The listing builds one solid part. Answer for the finished solid, in the listing's coordinates (mm). Coordinates: 2 decimals unless noted, no trailing zeros. Order: outer loops, then holes, each group sorted by start corner. A loop starts at its lowest first (then second) coordinate and runs counter-clockwise, first axis right, second up.
Autodesk Inventor part; units mm, degrees
ref_plane "YZ Plane" through (0, 0, 0) normal (1, 0, 0) x (0, 1, 0)
ref_plane "XZ Plane" through (0, 0, 0) normal (0, 1, 0) x (-1, 0, 0)
ref_plane "XY Plane" through (0, 0, 0) normal (0, 0, 1) x (1, 0, 0)
sketch "Sketch1" plane through (0, 0, 0) normal (1, 0, 0) x (0, 1, 0)
  line L0 (0, 0) -> (3, 0)
  line L1 (3, 0) -> (3, -87.28)
  line L2 (3, -87.28) -> (0, -87.28)
  line L3 (0, -87.28) -> (0, 0)
  line L4 (3.125, -87.405) -> (3.125, 0.125)
  line L5 (3.125, 0.125) -> (-0.125, 0.125)
  line L6 (-0.125, 0.125) -> (-0.125, -87.405)
  line L7 (-0.125, -87.405) -> (3.125, -87.405)
  line L8 (5.125, 2.125) -> (5.125, -89.405)
  line L9 (5.125, -89.405) -> (-2.125, -89.405)
  line L10 (-2.125, -89.405) -> (-2.125, 2.125)
  line L11 (-2.125, 2.125) -> (5.125, 2.125)
  line L12 (3, -87.28) -> (15, -87.28)
  line L13 (15, -87.28) -> (15, -84.28)
  line L14 (15, -84.28) -> (3, -84.28)
  line L15 (3, -84.28) -> (3, -87.28)
  line L16 (3, 0) -> (15, 0)
  line L17 (15, 0) -> (15, -3)
  line L18 (15, -3) -> (3, -3)
  line L19 (3, -3) -> (3, 0)
  line L20 (15.1, 0.1) -> (2.9, 0.1)
  line L21 (2.9, 0.1) -> (2.9, -3.1)
  line L22 (2.9, -3.1) -> (15.1, -3.1)
  line L23 (15.1, -3.1) -> (15.1, 0.1)
  line L24 (15.1, -87.38) -> (2.9, -87.38)
  line L25 (2.9, -87.38) -> (2.9, -84.18)
  line L26 (2.9, -84.18) -> (15.1, -84.18)
  line L27 (15.1, -84.18) -> (15.1, -87.38)
  line L28 (0.875, -89.405) -> (17.125, -89.405)
  line L29 (17.125, -89.405) -> (17.125, -82.155)
  line L30 (17.125, -82.155) -> (0.875, -82.155)
  line L31 (0.875, -82.155) -> (0.875, -89.405)
  line L32 (17.125, 2.125) -> (0.875, 2.125)
  line L33 (0.875, 2.125) -> (0.875, -5.125)
  line L34 (0.875, -5.125) -> (17.125, -5.125)
  line L35 (17.125, -5.125) -> (17.125, 2.125)
  line L36 (15.1, 0.1) -> (17.125, 0.1)
  line L37 (15.1, -3.1) -> (17.125, -3.1)
  line L38 (15.1, -87.38) -> (17.125, -87.38)
  line L39 (15.1, -84.18) -> (17.125, -84.18)
  point P0 (5.125, -82.155)
  point P1 (5.125, -5.125)
  point P2 (3.125, -84.18)
  point P3 (3.125, -87.38)
  point P4 (3.125, 0.1)
  point P5 (3.125, -3.1)
  dimension "d0" = 87.28
  dimension "d1" = 3
  dimension "d2" = 0.125
  dimension "d3" = 2
  dimension "d4" = 12
  dimension "d5" = 3
  dimension "d6" = 12
  dimension "d7" = 3
  dimension "d8" = 0.1
  dimension "d9" = 0.1
  dimension "d10" = 0
  dimension "d11" = 0
extrude "Extrusion1" add sketch "Sketch1" along normal blind 6.5 contours L33 L11 L8 L20 L4 L5 | L5 L6 L7 L31 L9 L10 L11 L33 | L7 L4 L24 L8 L9 L31 | L32 L35 L36 L20 L8 | L34 L8 L30 L4 | L4 L22 L8 L34 | L30 L8 L26 L4 | L8 L22 L37 L35 L34 | L8 L24 L38 L29 L28 | L30 L29 L39 L26 L8
sketch "Sketch2" plane through (6.5, 0, 0) normal (1, 0, 0) x (0, 0, -1)
  line L0 (3.1, 16.125) -> (-0.1, 16.125)
  line L1 (-0.1, 16.125) -> (-0.1, 3.325)
  line L2 (-0.1, 3.325) -> (3.1, 3.325)
  line L3 (3.1, 3.325) -> (3.1, 16.125)
  line L4 (3.1, 3.125) -> (84.18, 3.125)
  line L5 (5.125, 17.125) -> (3.1, 17.125)
  line L6 (-0.1, 3.125) -> (-0.1, 17.125)
  line L7 (3.1, 17.125) -> (3.1, 3.125)
  line L8 (84.18, 3.325) -> (87.38, 3.325)
  line L9 (87.38, 3.325) -> (87.38, 16.125)
  line L10 (87.38, 16.125) -> (84.18, 16.125)
  line L11 (84.18, 16.125) -> (84.18, 3.325)
  line L12 (89.405, 17.125) -> (87.38, 17.125)
  line L13 (87.38, 17.125) -> (87.38, 3.125)
  line L14 (84.18, 3.125) -> (84.18, 17.125)
  line L15 (28.765, -0.125) -> (58.515, -0.125)
  line L16 (58.515, -0.125) -> (58.515, 3.125)
  line L17 (58.515, 3.125) -> (28.765, 3.125)
  line L18 (28.765, 3.125) -> (28.765, -0.125)
  line L19 (87.405, -0.125) -> (-0.125, -0.125)
  line L20 (-0.125, -0.125) -> (-0.125, 3.125)
  point P0 (0, 0)
  dimension "d14" = 0.2
  dimension "d15" = 1
  dimension "d16" = 0
  dimension "d17" = 0
  dimension "d18" = 0.2
  dimension "d19" = 1
  dimension "d20" = 0
  dimension "d21" = 0
  dimension "d22" = 29.75
  dimension "d23" = 0
  dimension "d24" = 0
  dimension "d25" = 28.89
extrude "Extrusion2" add sketch "Sketch2" against normal blind 2.85
sketch "Sketch3" plane through (6.5, 0, 0) normal (1, 0, 0) x (0, 0, -1)
  line L0 (84.18, 16.125) -> (84.18, 17.125)
  line L1 (84.18, 17.125) -> (82.155, 17.125)
  line L2 (82.155, 17.125) -> (82.155, 5.125)
  line L3 (82.155, 5.125) -> (5.125, 5.125)
  line L4 (5.125, 5.125) -> (5.125, 17.125)
  line L5 (5.125, 17.125) -> (3.1, 17.125)
  line L6 (3.1, 17.125) -> (3.1, 16.125)
  line L7 (3.1, 16.125) -> (-0.1, 16.125)
  line L8 (-0.1, 16.125) -> (-0.1, 17.125)
  line L9 (-0.1, 17.125) -> (-2.125, 17.125)
  line L10 (-2.125, 17.125) -> (-2.125, -2.125)
  line L11 (-2.125, -2.125) -> (89.405, -2.125)
  line L12 (89.405, -2.125) -> (89.405, 17.125)
  line L13 (89.405, 17.125) -> (87.38, 17.125)
  line L14 (87.38, 17.125) -> (87.38, 16.125)
  line L15 (87.38, 16.125) -> (84.18, 16.125)
  line L16 (84.18, 3.325) -> (87.38, 3.325)
  line L17 (87.38, 3.325) -> (87.38, 3.125)
  line L18 (87.38, 3.125) -> (87.405, 3.125)
  line L19 (87.405, 3.125) -> (87.405, -0.125)
  line L20 (87.405, -0.125) -> (58.515, -0.125)
  line L21 (58.515, -0.125) -> (58.515, 3.125)
  line L22 (58.515, 3.125) -> (84.18, 3.125)
  line L23 (84.18, 3.125) -> (84.18, 3.325)
  line L24 (28.765, 3.125) -> (28.765, -0.125)
  line L25 (28.765, -0.125) -> (-0.125, -0.125)
  line L26 (-0.125, -0.125) -> (-0.125, 3.125)
  line L27 (-0.125, 3.125) -> (-0.1, 3.125)
  line L28 (-0.1, 3.125) -> (-0.1, 3.325)
  line L29 (-0.1, 3.325) -> (3.1, 3.325)
  line L30 (3.1, 3.325) -> (3.1, 3.125)
  line L31 (3.1, 3.125) -> (28.765, 3.125)
  point P0 (0, 0)
extrude "Extrusion4" add sketch "Sketch3" along normal blind 2.5 contours L15 L14 L13 L12 L11 L10 L9 L8 L7 L6 L5 L4 L3 L2 L1 L0 | L16 L17 L18 L19 L20 L21 L22 L23 | L24 L25 L26 L27 L28 L29 L30 L31
sketch "Sketch4" plane through (0, 0, 0) normal (-1, 0, 0) x (0, 0, 1)
  line L0 (-5.125, 5.125) -> (-5.125, 17.125)
  line L1 (-82.155, 17.125) -> (-82.155, 5.125)
  line L2 (-5.125, 5.125) -> (-82.155, 5.125)
  line L3 (-82.155, 5.125) -> (-82.155, 17.125)
  line L4 (-82.155, 17.125) -> (-5.125, 17.125)
  line L5 (-5.125, 17.125) -> (-5.125, 5.125)
  point P0 (0, 0)
extrude "Extrusion5" add sketch "Sketch4" against normal up to surface (9 mm away)
fillet "Fillet1" radius 1.25 2 edges at (4.5, -2.125, 2.125) (4.5, -2.125, -89.405)
properties part number "Front"
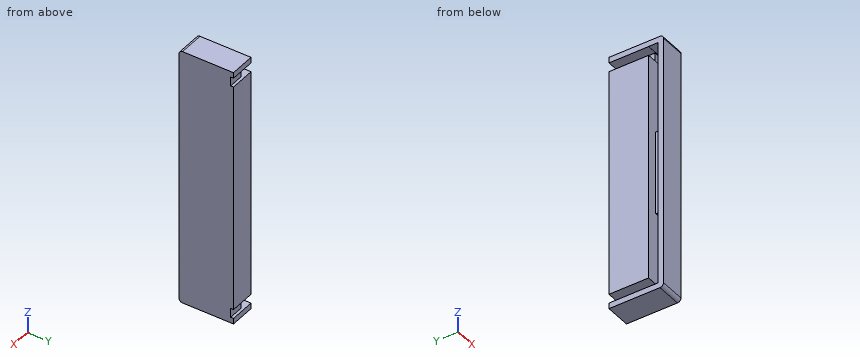
(1) This flat-tipped pin is pushed along its axis until it touches: pin 1 Ø1.6 at (y, z) = (11.5, -2) entering from -X. Where does it stop, or does it pass through?
(2) Consider line 1 (Z direction, x = 2.25, y = 16) (3 decimals); line 2 (Y direction, x = 4.25, z = -26) (3 decimals); line 3 (Z direction, x = 1.5, y = 0) (3 decimals). Determine where each line is inside the solid, lowest interval first.
(3) Find section D-D (x = 5.5). Give the number of separate pieces and of enclosed holes in the cut face, and give its area (3 significant figures).
(4) Find section B-B (z = -34). Write down the section's boundary in (x, y) (3 decimals), and give its area (3 significant figures).
(5) Find section A-A (x = 1.5). Write down the section's boundary in (y, z) (3 decimals), and give its area (3 significant figures).
(6) Find section C-C (y = 1.25). Write down the section's boundary in (x, z) (3 decimals).
Findings below:
1. pin 1: stops at x = 3.65
2. line 1: z = -89.405 to -87.38, -84.18 to -3.1, 0.1 to 2.125
2. line 2: y = -2.125 to -0.125, 3.125 to 17.125
2. line 3: z = -89.405 to -87.405, 0.125 to 2.125
3. separate pieces: 1
3. enclosed holes: 2
3. area: 1,570 mm2
4. outline: (0, -2.125) - (9, -2.125) - (9, 17.125) - (0, 17.125) - (0, 3.125) - (3.65, 3.125) - (3.65, -0.125) - (0, -0.125) - close
4. area: 161 mm2
5. outline: (-2.125, -88.155) arc R1.25 ccw to (-0.875, -89.405) - (17.125, -89.405) - (17.125, -87.38) - (3.125, -87.38) - (3.125, -87.405) - (-0.125, -87.405) - (-0.125, 0.125) - (3.125, 0.125) - (3.125, 0.1) - (17.125, 0.1) - (17.125, 2.125) - (-0.875, 2.125) arc R1.25 ccw to (-2.125, 0.875) - close; (3.125, -84.18) - (17.125, -84.18) - (17.125, -3.1) - (3.125, -3.1) - close
5. area: 1,390 mm2
6. outline: (0, -89.405) - (9, -89.405) - (9, 2.125) - (0, 2.125) - (0, 0.125) - (6.5, 0.125) - (6.5, -28.765) - (3.65, -28.765) - (3.65, -58.515) - (6.5, -58.515) - (6.5, -87.405) - (0, -87.405) - close
